Source: CAD feature listing. Evaluate the final solid. Frame: model axes, mm. A direction names the side the tool comes from. Give positions to 0.01 mm unless a question says otherwise; leave off trailing zeros. Write each loop counter-clockwise with the first axis right and the second up, starting at its lowest first coordinate (ties: lowest second). Pieces come first, ordered by that corner, then holes. Notation, with made-up numbers: (56.25, 67.5) -> (71.25, 67.5) arc R17 cw to (71.25, 97.5) -> close; hole circle Ø2 at (33.5, 38.25). An arc over 180 degrees is marked (long way). Write item = value, one per line.
from build123d import *

# Parameters (mm, degrees)
F1_DEPTH    = 80
F0_W        = 20.5
F0_H        = 15
F0_W_2      = 5.5
F2_DEPTH    = 30
F0_W_3      = 15
F3_DEPTH    = 20
F4_T1_DEPTH = 123.2356797549
F4_T3_DEPTH = 123.2356797549
F5_T1_DEPTH = 164.157613302
F6_R        = 10
F7_R        = 2
F8_R        = 3


# Not quite as in the source:
# - a fillet or chamfer that OpenCascade refuses, or shapes differently, is made with other operations: its cross-section is extruded or revolved along the edge and cut away or added


with BuildPart() as f1:
    # F0 (on Front) → F1 (new body)
    with BuildSketch(Plane.XZ):
        with BuildLine():
            Line((-20.5, 15), (-38.75, 15))
            Line((-38.75, 15), (-38.75, 10.0617376915))
            ThreePointArc((-38.75, 10.0617376915), (-36.1987907943, 9.7707377656), (-35, 7.5))
            ThreePointArc((-35, 7.5), (-36.1987907943, 5.2292622344), (-38.75, 4.9382623085))
            Line((-38.75, 4.9382623085), (-38.75, 0))
            Line((-38.75, 0), (-20.5, 0))
            Line((-20.5, 0), (-20.5, 15))
        make_face()
    extrude(amount=F1_DEPTH)

    # F0 (on Front) → F2 (join)
    with BuildSketch(Plane.XZ):
        with Locations((-10.25, 7.5)):
            Rectangle(F0_W, F0_H)
        with Locations((2.75, 7.5)):
            Rectangle(F0_W_2, F0_H)
    extrude(amount=F2_DEPTH)



with BuildPart() as f1b:
    # F0 (on Front) → F1, piece 2 (new body)
    with BuildSketch(Plane.XZ):
        with BuildLine():
            Line((38.75, 15), (20.5, 15))
            Line((20.5, 15), (20.5, 0))
            Line((20.5, 0), (38.75, 0))
            Line((38.75, 0), (38.75, 4.9382623085))
            ThreePointArc((38.75, 4.9382623085), (35, 7.5), (38.75, 10.0617376915))
            Line((38.75, 10.0617376915), (38.75, 15))
        make_face()
        with BuildLine():
            Line((44.75, 15), (38.75, 15))
            Line((38.75, 15), (38.75, 10.0617376915))
            ThreePointArc((38.75, 10.0617376915), (40.0207377656, 9.0512092057), (40.5, 7.5))
            ThreePointArc((40.5, 7.5), (40.0207377656, 5.9487907943), (38.75, 4.9382623085))
            Line((38.75, 4.9382623085), (38.75, 0))
            Line((38.75, 0), (44.75, 0))
            Line((44.75, 0), (44.75, 15))
        make_face()
    extrude(amount=F1_DEPTH)


with BuildPart() as f1_1:
    add(f1.part)

    add(f1b.part)  # F3 merges F1b
    # F0 (on Front) → F3 (join)
    with BuildSketch(Plane.XZ):
        with Locations((13, 7.5)):
            Rectangle(F0_W_3, F0_H)
    extrude(amount=F3_DEPTH)

    # F4: chamfer of 23 on 2 edges, made by hand

    # F4_s2 → F4_t1 (cut)
    with BuildSketch(Plane.XY.offset(-59.1487087232)):
        Polygon((-15.75, 0), (-38.75, -23), (-38.75, 0), align=None)
    extrude(amount=F4_T1_DEPTH, mode=Mode.SUBTRACT)

    # F4_s4 → F4_t3 (cut)
    with BuildSketch(Plane.XY.offset(-49.0869710317)):
        Polygon((-15.75, 0), (-38.75, -23), (-38.75, 0), align=None)
    extrude(amount=F4_T3_DEPTH, mode=Mode.SUBTRACT)

    # F5: chamfer of 29 on 1 edges, made by hand

    # F5_s2 → F5_t1 (cut)
    with BuildSketch(Plane.XY.offset(-74.578806651)):
        Polygon((15.75, 0), (44.75, -29), (44.75, 0), align=None)
    extrude(amount=F5_T1_DEPTH, mode=Mode.SUBTRACT)

    # F6
    f6_edges = [f1_1.edges().sort_by_distance(p)[0] for p in [
        (15.75, 0, 7.5),
        (-15.75, 0, 7.5),
        (44.75, -29, 7.5),
        (-38.75, -23, 2.469131),
        (-38.75, -23, 12.530869),
    ]]
    fillet(f6_edges, radius=F6_R)

    # F7
    f7_edges = [f1_1.edges().sort_by_distance(p)[0] for p in [
        (20.5, -50, 15),
        (20.5, -50, 0),
        (-20.5, -55, 15),
        (-20.5, -55, 0),
        (5.5, -30, 7.5),
    ]]
    fillet(f7_edges, radius=F7_R)

    # F8
    f8_edges = [f1_1.edges().sort_by_distance(p)[0] for p in [
        (-38.75, -53.571068, 15),
        (-37.988795, -23.315301, 15),
        (-27.25, -11.5, 15),
        (-15.434699, -0.761205, 15),
        (0, 0, 15),
        (15.434699, -0.761205, 15),
        (30.25, -14.5, 15),
        (43.988795, -29.315301, 15),
        (44.75, -56.571068, 15),
        (44.75, -56.571068, 0),
        (43.988795, -29.315301, 0),
        (-38.75, -53.571068, 0),
        (-37.988795, -23.315301, 0),
        (-27.25, -11.5, 0),
        (-15.434699, -0.761205, 0),
        (0, 0, 0),
        (15.434699, -0.761205, 0),
        (30.25, -14.5, 0),
    ]]
    fillet(f8_edges, radius=F8_R)


solid = f1_1.part
(1) Access query for faces 1 (the face through (-20.5, -55, 7)), 2 (the face through (44.75, -56, 7)), 3 (the face through (-21.07, -55.35, 14.4)). Directions: +Z, -Z, +X, -X, +Y, -Y. A direction counts if a zero-diameter tool reaches every point of the face in a straight line with its end or side. Return the directions, or none.
Values follow:
face_1 = +Z, -Z, -Y
face_2 = +Z, -Z, +X, +Y, -Y
face_3 = +Z, -Y
(2) First-contact query: pin 1 (7.5 mm diameter, centred on x = -10.5, z = 11, fed in from -Y); pin 2 (10 mm diameter, centred on x = -29.5, y = -8.5, fed in from -Z); pin 3 (4 mm diameter, centred on y = -25, z = 10.5, fed in from +X). Flat tips, straight axial feed; report the tip coordinate or a pass-through.
Values follow:
pin_1 = -30
pin_2 = 0.54
pin_3 = 42.64
(3) Material intervals for line 1 (X direction, y = -53, z = 7.5); line 2 (Z direction, x = 37.75, y = -41); line 3 (X direction, y = -41, z = 8.75), sorted ascending.
Values follow:
line_1 = -35 to -20.5, 20.5 to 35, 40.5 to 44.75
line_2 = 0 to 4.75, 10.25 to 15
line_3 = -35.3 to -20.5, 20.5 to 35.3, 40.2 to 44.75
(4) Pull-direction query (X, two-part tool) for faces 4 (the face through (-37.85, -53.2, 0.86)), 5 (the face through (43.85, -56.9, 0.86)), 6 (the face through (-21.1, -55.35, 0.57)), 7 (the face through (20.5, -50, 8)); classes: pulls with the +X half, pulls with the -X half, needs draft (parallel to the pull), parting line crosses it, or undercut.
Values follow:
face_4 = pulls with the -X half
face_5 = pulls with the +X half
face_6 = undercut
face_7 = undercut
(5) Section query A-A (y = -49). Return loops of the section in (x, z).
Values follow:
outline = (-38.75, 3) arc R3 ccw to (-35.75, 0) -> (-22.5, 0) arc R2 ccw to (-20.5, 2) -> (-20.5, 13) arc R2 ccw to (-22.5, 15) -> (-35.75, 15) arc R3 ccw to (-38.75, 12) -> (-38.75, 10.06) arc R2.75 cw (long way) to (-38.75, 4.94) -> close; (20.5, 2) arc R2 ccw to (22.5, 0) -> (41.75, 0) arc R3 ccw to (44.75, 3) -> (44.75, 12) arc R3 ccw to (41.75, 15) -> (22.5, 15) arc R2 ccw to (20.5, 13) -> close; hole circle Ø5.5 at (37.75, 7.5)
